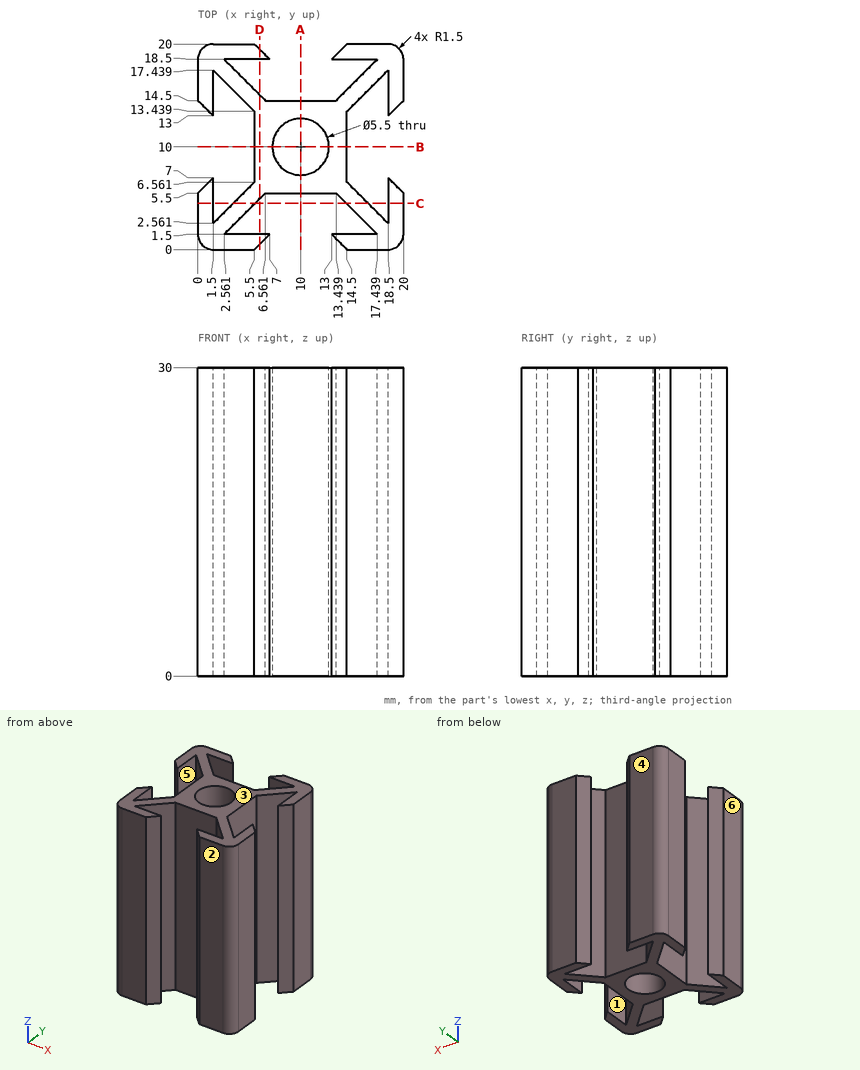
Here's the drawing with two shaded views (mm, measured from the low corner). I have some questions. A direction names the side the tool comes from. Coordinates: 2 decimals unless noted, no trailing zeros. Write each loop counter-clockwise with the first axis right and the second up, starting at its lowest first coordinate (ties: lowest second). Pieces come first, ordered by that corner, then holes. Notation, with made-up numbers: M 21.25,-7 L 36.25,-7 A13 cw 36.25,10 Z; hole C 55.25,0.25 d1. An arc over 180 degrees is marked long. Write item = value, one per line. Start each with the question number.
Q1. If we section it at C-C, the plane y = 4.5: Write out the boundary of the cut face in (x, z).
Q2. I'm going to push flat-ended pins straight in: pin 1 (2 mm diameter, centred on x = 10.5, z = 14.5, fed in from -Y); pin 2 (5.5 mm diameter, centred on x = 10, z = 10, fed in from +Y); pin 3 (2 mm diameter, centred on y = 10, z = 8, fed in from +X); pin 4 (3.5 mm diameter, centred on x = 10, y = 10, fed in from +Z). Where does each tip first touch, or does it pass through?
Q3. If I drill on L1, parallel to X at y = 3, z = 20.75; L2, parallel to Y at x = 10, z = 14.5; L3, parallel to X at y = 5, z = 20, over which ranges is the centre line in solid material (lowest first)? Write a range as [from, to].
Q4. Thinking about a two-plate mould opening in Y: for the marked faces 1, 2, 3 and 4, which applies, released by +Y, released by -Y, zero draft, split by the parting line, or undercut?
Q5. On a 3-axis mill with a long thin cutter (end or side, diameter ignored), from which of +Z, -Z, +X, -X, +Y, -Y can I reach the whole of each face in a straight line? I mean the marked faces 5 and 6. Say none if no direction works.
Q6. If we section it at A-A, the plane x = 10: Write out the boundary of the cut face in (y, z).
Q7. If we section it at D-D, the plane x = 6: Write out the boundary of the cut face in (y, z).
Check sheet entries:
q1.outline = M 0,0 L 1.5,0 L 1.5,30 L 0,30 Z; M 3.44,0 L 5.56,0 L 5.56,30 L 3.44,30 Z; M 14.44,0 L 16.56,0 L 16.56,30 L 14.44,30 Z; M 18.5,0 L 20,0 L 20,30 L 18.5,30 Z
q2.pin_1 = 5.5
q2.pin_2 = 14.5
q2.pin_3 = 14.5
q2.pin_4 = through
q3.L1 = [0, 1.5], [1.94, 4.06], [15.94, 18.06], [18.5, 20]
q3.L2 = [5.5, 7.25], [12.75, 14.5]
q3.L3 = [0, 1.5], [3.94, 6.06], [13.94, 16.06], [18.5, 20]
q4.face_1 = undercut
q4.face_2 = released by -Y
q4.face_3 = zero draft
q4.face_4 = released by +Y
q5.face_5 = +Z, -Z
q5.face_6 = +Z, -Z, -X, +Y, -Y
q6.outline = M 5.5,0 L 7.25,0 L 7.25,30 L 5.5,30 Z; M 12.75,0 L 14.5,0 L 14.5,30 L 12.75,30 Z
q7.outline = M 0.5,0 L 1.5,0 L 1.5,30 L 0.5,30 Z; M 4.94,0 L 15.06,0 L 15.06,30 L 4.94,30 Z; M 18.5,0 L 19.5,0 L 19.5,30 L 18.5,30 Z
